from build123d import *

# Parameters (mm, degrees)
SKETCH4_R          = 7.7597
SKETCH4_R_2        = 7.60095
CUT_EXTRUDE2_DEPTH = 7.112
CUT_EXTRUDE1_DEPTH = 7.112
CIRPATTERN1_COUNT  = 24
SKETCH6_R          = 3
CUT_EXTRUDE3_DEPTH = 23.397327676


with BuildPart() as part:
    # Sketch1 → Revolve1 (revolve)
    with BuildSketch(Plane.XY, mode=Mode.PRIVATE) as revolve1_sk:
        with BuildLine():
            Line((-8.7376, 2.38125), (8.7376, 2.38125))
            Line((8.7376, 2.38125), (8.7376, 9.906))
            Line((8.7376, 9.906), (7.7343, 9.906))
            ThreePointArc((7.7343, 9.906), (7.003135774, 9.264822773), (6.731, 8.3312))
            Line((6.731, 8.3312), (6.731, 7.7597))
            Line((6.731, 7.7597), (-0.381, 7.7597))
            Line((-0.381, 7.7597), (-0.381, 8.3312))
            ThreePointArc((-0.381, 8.3312), (-0.653135774, 9.264822773), (-1.3843, 9.906))
            Line((-1.3843, 9.906), (-2.3876, 9.906))
            Line((-2.3876, 9.906), (-2.3876, 6.35))
            Line((-2.3876, 6.35), (-8.7376, 6.35))
            Line((-8.7376, 6.35), (-8.7376, 2.38125))
        make_face()
    revolve(revolve1_sk.sketch.rotate(Axis((-8.7376, 0, 0), (1, 0, 0)), 90), axis=Axis((-8.7376, 0, 0), (1, 0, 0)))

    # Sketch4 → Cut-Extrude2 (cut)
    with BuildSketch(Plane(origin=(-0.381, 0, 0), x_dir=(0, 0, -1), z_dir=(1, 0, 0))):
        Circle(SKETCH4_R)
        with Locations(Location((0, 0, 0), (0, 0, 180))):
            Circle(SKETCH4_R_2, mode=Mode.SUBTRACT)
    extrude(amount=CUT_EXTRUDE2_DEPTH, mode=Mode.SUBTRACT)

    # Sketch3 → Cut-Extrude1 (cut)
    with BuildSketch(Plane(origin=(-0.381, 0, 0), x_dir=(0, 0, -1), z_dir=(1, 0, 0))):
        with BuildLine():
            Line((-0.643066132, 7.57369836), (-0.340952079, 6.925812683))
            Line((-0.340952079, 6.925812683), (0.340952079, 6.925812683))
            Line((0.340952079, 6.925812683), (0.643066132, 7.57369836))
            ThreePointArc((0.643066132, 7.57369836), (0, 7.60095), (-0.643066132, 7.57369836))
        make_face()
    cut_extrude1 = extrude(amount=CUT_EXTRUDE1_DEPTH, mode=Mode.SUBTRACT)

    # CirPattern1: Cut-Extrude1 ×24 about axis
    cirpattern1_axis = Axis((0, 0, 0), (1, 0, 0))
    for i in range(1, CIRPATTERN1_COUNT):
        add(cut_extrude1.rotate(cirpattern1_axis, i * 360 / CIRPATTERN1_COUNT), mode=Mode.SUBTRACT)

    # Sketch6 → Cut-Extrude3 (cut, through all)
    with BuildSketch(Plane.ZY.offset(8.7376)):
        Circle(SKETCH6_R)
    extrude(amount=-CUT_EXTRUDE3_DEPTH, mode=Mode.SUBTRACT)


solid = part.part
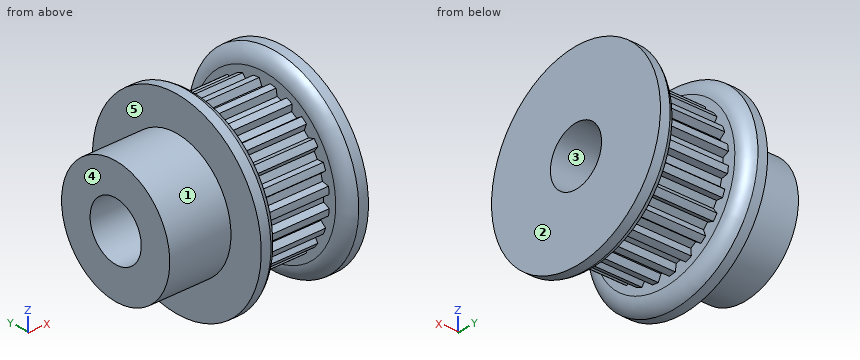
Model file for the job. Use its own axes, mm. Face numbers are marked on the shaded views. A direction names the side the tool comes from. Coordinates: 2 decimals unless noted, no trailing zeros. Order: outer loops, then holes, each group sorted by start corner. A loop starts at its lowest first (then second) coordinate and runs counter-clockwise, first axis right, second up. Notation, with made-up numbers: (-15, 47.25) -> (18, 47.25) arc R6 cw to (18, 55.25) -> close; hole circle Ø5 at (-34.5, -24.5). An arc over 180 degrees is marked (long way). Return JSON: item names as keys, results as strings. Group by question number.
Item 1: Pull direction Y, two halves, no side cores. Call the marked faces 1, 2 and 3: pulls with the +Y half, pulls with the -Y half, needs draft (parallel to the pull), parting line crosses it, or undercut.
Item 2: Flat gauge pins, fed straight in: P1, Ø4, axis at x = -5.5, z = -2, coming from the -Y side; P2, Ø1.5, axis at x = -6, y = -2, coming from the +Z side. Where does each tip first touch, or does it go through?
Item 3: Wall check: line 1 along X through (y, z) = (-5, 6); line 2 along Z through (x, y) = (2.25, -6); line 3 along Y through (x, z) = (-3.5, 0). Give the ranges that are in metal, low to high. Write a range as [from, to].
Item 4: Saw through at A-A on z = 0. Write the cut outline in (x, y).
Item 5: Saw through at C-C on x = -7.5. Write the cut outline in (y, z), then the cut area to 3 significant figures.
Item 6: Saw through at D-D on x = -1. Write the cut outline in (y, z).
Item 7: Tool access for the marked faces 4 and 5: list every direction of +Z, -Z, +X, -X, +Y, -Y with a clear straight run to the whole face (end or side of a thin tool).
Values found:
{
 "1": {"face 1": "parting line crosses it", "face 2": "needs draft", "face 3": "undercut"},
 "2": {"P1": "stops at y = -6.35", "P2": "stops at z = 6.23"},
 "3": {"line 1": "x = [-2.39, -0.38], [6.73, 8.74]", "line 2": "z = [-4.67, -4], [-3.46, 3.46], [4, 4.67]", "line 3": "y = [-6.35, -3], [3, 6.35]"},
 "4": {"outline": "(-8.74, -6.35) -> (-2.39, -6.35) -> (-2.39, -9.91) -> (-1.38, -9.91) arc R1.74 ccw to (-0.38, -8.33) -> (-0.38, -6.93) -> (6.73, -6.93) -> (6.73, -8.33) arc R1.74 ccw to (7.73, -9.91) -> (8.74, -9.91) -> (8.74, -3) -> (-8.74, -3) -> close; (-8.74, 3) -> (8.74, 3) -> (8.74, 9.91) -> (7.73, 9.91) arc R1.74 ccw to (6.73, 8.33) -> (6.73, 6.93) -> (-0.38, 6.93) -> (-0.38, 8.33) arc R1.74 ccw to (-1.38, 9.91) -> (-2.39, 9.91) -> (-2.39, 6.35) -> (-8.74, 6.35) -> close"},
 "5": {"outline": "circle Ø12.7 at (0, 0); hole circle Ø6 at (0, 0)", "area": "98.4 mm2"},
 "6": {"outline": "circle Ø19.32 at (0, 0); hole circle Ø6 at (0, 0)"},
 "7": {"face 4": "+Z, -Z, -X, +Y, -Y", "face 5": "-X"}
}
